Part print with two shaded views. Sizes in mm from the minimum x, y, z corner. A direction names the side the tool comes from. Coordinates: 2 decimals unless noted, no trailing zeros. Loops run counter-clockwise (first coordinate to the right, second up) from the corner with the lowest first, then second, coordinate; pieces in that order, holes last. Notation, with made-up numbers: (41, -22.5) -> (98, -22.5) arc R23 cw to (98, 5.5) -> close; hole circle Ø2 at (10.5, -8.5). An arc over 180 degrees is marked (long way). Return JSON: item names as keys, results as strings. Group by question number.
(1) Saw through at C-C on z = 7.5. Write the cut outline in (x, y).
(2) Saw through at A-A on x = 39.5. Write the cut outline in (y, z).
(3) Mould opens along Y. For the marked faces 1, 2 and 3 say: pulls with the +Y half, pulls with the -Y half, needs draft (parallel to the pull), parting line crosses it, or undercut.
(4) Probe L1, parallel to X at y = 7.5, z = 61.25; L2, parallel to X at y = 7.5, z = 41.75; L3, parallel to X at y = 7.75, z = 13.5. List the from-to ranges inside material, lowest first.
(5) Saw through at D-D on y = 2.75. Write the cut outline in (x, z).
(6) Saw through at B-B on y = 7.5. Write the cut outline in (x, z), then the cut area to 3 significant figures.
(7) Flat gauge pins, fed straight in: pin 1 Ø1 at (y, z) = (6.5, 12.5) entering from -X; pin 2 Ø4 at (x, y) = (39.5, 8) entering from -Z; pin 3 Ø3 at (x, y) = (16, 4) entering from -Z; pin 4 Ø5 at (x, y) = (39.5, 7.5) entering from +Z. Where does each tip first touch, or does it go through?
(8) Tool access for the marked faces 4 and 5: list every direction of +Z, -Z, +X, -X, +Y, -Y with a clear straight run to the whole face (end or side of a thin tool).
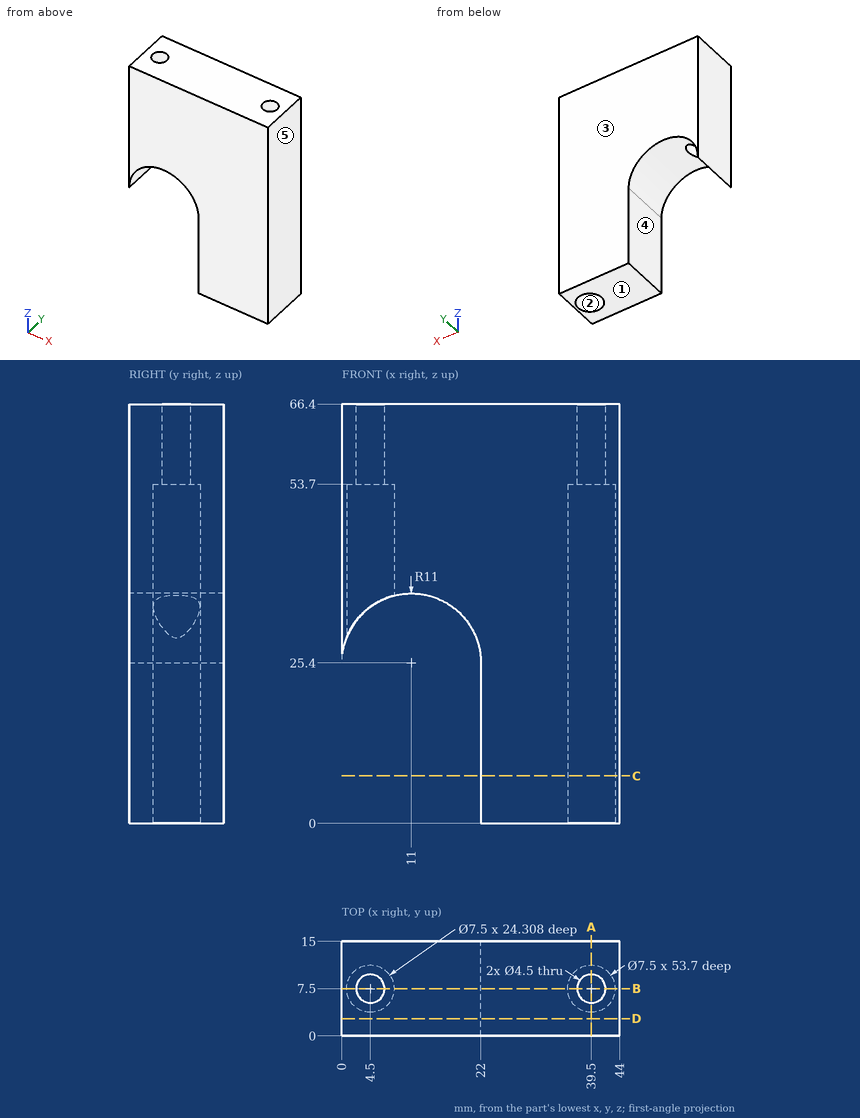
Geometry results:
{
 "1": {"outline": "(22, 0) -> (44, 0) -> (44, 15) -> (22, 15) -> close; hole circle Ø7.5 at (39.5, 7.5)"},
 "2": {"outline": "(0, 0) -> (3.75, 0) -> (3.75, 53.7) -> (5.25, 53.7) -> (5.25, 66.4) -> (0, 66.4) -> close; (9.75, 53.7) -> (11.25, 53.7) -> (11.25, 0) -> (15, 0) -> (15, 66.4) -> (9.75, 66.4) -> close"},
 "3": {"face 1": "needs draft", "face 2": "undercut", "face 3": "pulls with the +Y half"},
 "4": {"L1": "0 to 2.25, 6.75 to 37.25, 41.75 to 44", "L2": "0 to 0.75, 8.25 to 35.75, 43.25 to 44", "L3": "22 to 35.76, 43.24 to 44"},
 "5": {"outline": "(0, 25.4) arc R11 cw to (22, 25.4) -> (22, 0) -> (44, 0) -> (44, 66.4) -> (0, 66.4) -> close"},
 "6": {"outline": "(0, 25.4) arc R11 cw to (0.75, 29.39) -> (0.75, 53.7) -> (2.25, 53.7) -> (2.25, 66.4) -> (0, 66.4) -> close; (6.75, 53.7) -> (8.25, 53.7) -> (8.25, 36.05) arc R11 cw to (22, 25.4) -> (22, 0) -> (35.75, 0) -> (35.75, 53.7) -> (37.25, 53.7) -> (37.25, 66.4) -> (6.75, 66.4) -> close; (41.75, 53.7) -> (43.25, 53.7) -> (43.25, 0) -> (44, 0) -> (44, 66.4) -> (41.75, 66.4) -> close", "area": "1,510 mm²"},
 "7": {"pin 1": "x = 22", "pin 2": "z = 53.7", "pin 3": "z = 34.27", "pin 4": "z = 66.4"},
 "8": {"face 4": "-Z, -X, +Y, -Y", "face 5": "+Z, -Z, +X, +Y, -Y"}
}
